from build123d import *

# Parameters (mm, degrees)
CROQUIS1_W              = 10
CROQUIS1_H              = 25
SALIENTE_EXTRUIR1_DEPTH = 5
CROQUIS2_R              = 1
SALIENTE_EXTRUIR2_DEPTH = 15


with BuildPart() as part:
    # Croquis1 → Saliente-Extruir1 (new body)
    with BuildSketch(Plane(origin=(0, 0, 0), x_dir=(1, 0, 0), z_dir=(0, 1, 0))):
        Rectangle(CROQUIS1_W, CROQUIS1_H)
    extrude(amount=SALIENTE_EXTRUIR1_DEPTH)

    # Croquis2 → Saliente-Extruir2 (add)
    with BuildSketch(Plane(origin=(0, 5, 0), x_dir=(1, 0, 0), z_dir=(0, 1, 0))):
        with Locations((0, 6.5)):
            Circle(CROQUIS2_R)
    extrude(amount=SALIENTE_EXTRUIR2_DEPTH)


solid = part.part
Source: CAD feature listing. Evaluate the final solid. Frame: model axes, mm. A direction names the side the tool comes from. Round coordinates to 2 decimals unless told otherwise and drop trailing zeros. Loops run counter-clockwise (first coordinate to the right, second up) from the corner with the lowest first, then second, coordinate; pieces in that order, holes last. Notation, with made-up numbers: (77.25, -1) -> (81.25, -1) arc R21 cw to (81.25, 36) -> close; hole circle Ø8 at (-5.75, 64). An arc over 180 degrees is marked (long way). Answer as a JSON object with one key per item and string values. Group by question number.
Q1. Section query A-A (x = 0). Output: boundary loops of the cut face in (y, z), plus the area to 3 significant figures.
Q2. Ray query, line 1 (Y direction, x = 3.5, z = -0.5); line 2 (Z direction, x = 0.75, y = 11.75); line 3 (X direction, y = 15.5, z = -7). Return the intervals inside material, ascending. Write a range as from..to.
Q3. Section query C-C (y = 6.5). Output: boundary loops of the cut face in (x, z), plus the area to 3 significant figures.
Q4. Access query for faces 1 (the cylindrical face through (-0.13, 12.4, -7.49)), 2 (the flat face through (5, 2, 0)). Directions: +Z, -Z, +X, -X, +Y, -Y. A direction counts if a zero-diameter tool reaches every point of the face in a straight line with its end or side. Return the directions, or none.
Q5. Contact query for flat-ended pins moving along their axis: P1, Ø6, axis at x = 2, z = 1, coming from the -Y side; P2, Ø6, axis at x = 0, z = 5.5, coming from the +Y side; P3, Ø6, axis at x = 0.5, y = 14, coming from the +Z side. Output: stop coordinate, or through.
Q6. Section query B-B (z = -6.5). Output: boundary loops of the cut face in (x, y).
Q7. Section query D-D (x = 2.75). Output: boundary loops of the cut face in (y, z), plus the area to 3 significant figures.
Completed:
{
 "1": {"outline": "(0, -12.5) -> (5, -12.5) -> (5, -7.5) -> (20, -7.5) -> (20, -5.5) -> (5, -5.5) -> (5, 12.5) -> (0, 12.5) -> close", "area": "155 mm²"},
 "2": {"line 1": "0..5", "line 2": "-7.16..-5.84", "line 3": "-0.87..0.87"},
 "3": {"outline": "circle Ø2 at (0, -6.5)", "area": "3.14 mm²"},
 "4": {"face 1": "+Y", "face 2": "+Z, -Z, +X, +Y, -Y"},
 "5": {"P1": "y = 0", "P2": "y = 5", "P3": "z = -5.5"},
 "6": {"outline": "(-5, 0) -> (5, 0) -> (5, 5) -> (1, 5) -> (1, 20) -> (-1, 20) -> (-1, 5) -> (-5, 5) -> close"},
 "7": {"outline": "(0, -12.5) -> (5, -12.5) -> (5, 12.5) -> (0, 12.5) -> close", "area": "125 mm²"}
}
